```python
from build123d import *

# Parameters (mm, degrees)
F1_DEPTH = 3


with BuildPart() as f1:
    # F0 (on Front) → F1 (new body)
    with BuildSketch(Plane.XZ):
        Polygon((-17.5, 110.7), (-17.5, 113.7), (-37.5, 113.7), (-37.5, 110.7), (-34.5, 110.7), (-34.5, 94.7), (-37.5, 94.7), (-37.5, 78.7), (-34.5, 78.7), (-34.5, 62.7), (-37.5, 62.7), (-37.5, 46.7), (-34.5, 46.7), (-34.5, 30.7), (-37.5, 30.7), (-37.5, 14.7), (-34.5, 14.7), (-34.5, -0.7), (-37.5, -0.7), (-37.5, -6.7), (-17.5, -6.7), (-17.5, -3.7), (2.5, -3.7), (2.5, -6.7), (22.5, -6.7), (22.5, -3.7), (42.5, -3.7), (42.5, -6.7), (62.5, -6.7), (62.5, -3.7), (77.5, -3.7), (77.5, -6.7), (82.5, -6.7), (82.5, -3.7), (97.5, -3.7), (97.5, -6.7), (117.5, -6.7), (117.5, -3.7), (137.5, -3.7), (137.5, -6.7), (157.5, -6.7), (157.5, -3.7), (177.5, -3.7), (177.5, -6.7), (197.5, -6.7), (197.5, -0.7), (194.5, -0.7), (194.5, 14.7), (197.5, 14.7), (197.5, 30.7), (194.5, 30.7), (194.5, 46.7), (197.5, 46.7), (197.5, 62.7), (194.5, 62.7), (194.5, 78.7), (197.5, 78.7), (197.5, 94.7), (194.5, 94.7), (194.5, 110.7), (197.5, 110.7), (197.5, 113.7), (177.5, 113.7), (177.5, 110.7), (157.5, 110.7), (157.5, 113.7), (137.5, 113.7), (137.5, 110.7), (117.5, 110.7), (117.5, 113.7), (97.5, 113.7), (97.5, 110.7), (82.5, 110.7), (82.5, 113.7), (77.5, 113.7), (77.5, 110.7), (62.5, 110.7), (62.5, 113.7), (42.5, 113.7), (42.5, 110.7), (22.5, 110.7), (22.5, 113.7), (2.5, 113.7), (2.5, 110.7), align=None)
        with BuildLine():
            Line((155, 0), (5, 0))
            ThreePointArc((5, 0), (1.464466, 1.464466), (0, 5))
            Line((0, 5), (0, 70))
            ThreePointArc((0, 70), (-0.87868, 72.12132), (-3, 73))
            Line((-3, 73), (-8, 73))
            ThreePointArc((-8, 73), (-13, 78), (-8, 83))
            Line((-8, 83), (-3, 83))
            ThreePointArc((-3, 83), (-0.87868, 83.87868), (0, 86))
            Line((0, 86), (0, 100))
            ThreePointArc((0, 100), (1.464466, 103.535534), (5, 105))
            Line((5, 105), (155, 105))
            ThreePointArc((155, 105), (158.535534, 103.535534), (160, 100))
            Line((160, 100), (160, 5))
            ThreePointArc((160, 5), (158.535534, 1.464466), (155, 0))
        make_face(mode=Mode.SUBTRACT)
    extrude(amount=-F1_DEPTH)


solid = f1.part
```
Source: CAD feature listing. Evaluate the final solid. Frame: model axes, mm. A direction names the side the tool comes from. Give positions to 0.01 mm unless a question says otherwise; leave off trailing zeros. Order: outer loops, then holes, each group sorted by start corner. A loop starts at its lowest first (then second) coordinate and runs counter-clockwise, first axis right, second up. Notation, with made-up numbers: (13.25, 42) -> (65.25, 42) arc R8 cw to (65.25, 51) -> close; hole circle Ø1 at (-36.5, 26). An arc over 180 degrees is marked (long way). Use a Markdown table: item, result.
Q1. Section B-B (z = 90). Return the cut outline in (x, y), and give its area (3 significant figures).
A:
| item | result |
|---|---|
| outline | (-37.5, 0) -> (0, 0) -> (0, 3) -> (-37.5, 3) -> close; (160, 0) -> (197.5, 0) -> (197.5, 3) -> (160, 3) -> close |
| area | 225 mm^2 |
Q2. Section A-A (x = 27). Return the cut outline in (y, z).
A:
| item | result |
|---|---|
| outline | (0, -3.7) -> (3, -3.7) -> (3, 0) -> (0, 0) -> close; (0, 105) -> (3, 105) -> (3, 110.7) -> (0, 110.7) -> close |
Q3. Pull-direction query (X, two-part tool) for faces 3 (the face through (71, 0, 107)), 4 (the face through (158, 1, 104)); classes: +X half, -X half, draft (parallel to the pull), parting line (faces both ways), or undercut.
A:
| item | result |
|---|---|
| face 3 | draft |
| face 4 | undercut |
Q4. Material intervals for line 1 (X direction, y = 0.7, z = 15.5); line 2 (Z direction, x = 119, y = 2.75); line 3 (Z direction, x = 141.5, y = 0.55), sorted ascending. Write a range as [from, to].
A:
| item | result |
|---|---|
| line 1 | [-37.5, 0], [160, 197.5] |
| line 2 | [-3.7, 0], [105, 110.7] |
| line 3 | [-6.7, 0], [105, 113.7] |
Q5. Access query for faces 1 (the face through (159, 1, 2)), 2 (the face through (71, 3, 107)). Directions: +Z, -Z, +X, -X, +Y, -Y. A direction counts if a zero-diameter tool reaches every point of the face in a straight line with its end or side. Return the directions, or none.
A:
| item | result |
|---|---|
| face 1 | +Y, -Y |
| face 2 | +Z, -Z, +X, -X, +Y |
Q6. Section C-C (x = 164.5). Return the cut outline in (y, z), and give its area (3 significant figures).
A:
| item | result |
|---|---|
| outline | (0, -3.7) -> (3, -3.7) -> (3, 110.7) -> (0, 110.7) -> close |
| area | 343 mm^2 |
Q7. First-contact query: P1, Ø0.9, axis at x = 129.5, y = 2, coming from the -Z side; P2, Ø1.5, axis at y = 1, z = 4.5, coming from the -X side. Flat tips, straight axial feed; report the tip coordinate or a pass-through.
A:
| item | result |
|---|---|
| P1 | z = -3.7 |
| P2 | x = -34.5 |
